from build123d import *

# Parameters (mm, degrees)
F0_R     = 11.5
F1_DEPTH = 11
F2_R     = 11.5
F3_DEPTH = 3
F6_DEPTH = 10


# Not quite as in the source:
# - a fillet or chamfer that OpenCascade refuses, or shapes differently, is made with other operations: its cross-section is extruded or revolved along the edge and cut away or added


with BuildPart() as f1:
    # F0 (on Top) → F1 (new body)
    with BuildSketch(Plane.XY):
        Circle(F0_R)
        Polygon((9.5, 1.5), (9.5, -1.5), (1.5, -1.5), (1.5, -9.5), (-1.5, -9.5), (-1.5, -1.5), (-9.5, -1.5), (-9.5, 1.5), (-1.5, 1.5), (-1.5, 9.5), (1.5, 9.5), (1.5, 1.5), align=None, mode=Mode.SUBTRACT)
    extrude(amount=F1_DEPTH)

    # F2 (on face) → F3 (join)
    with BuildSketch(Plane.XY.offset(11)):
        Circle(F2_R)
        Polygon((1.5, 1.5), (9.5, 1.5), (9.5, -1.5), (1.5, -1.5), (1.5, -9.5), (-1.5, -9.5), (-1.5, -1.5), (-9.5, -1.5), (-9.5, 1.5), (-1.5, 1.5), (-1.5, 9.5), (1.5, 9.5), align=None, mode=Mode.SUBTRACT)
    extrude(amount=F3_DEPTH)

    # F4: fillet of radius 5 on 1 edges, made by hand

    # F4_s1 → F4_t2 (revolve, cut)
    with BuildSketch(Plane.XZ):
        with BuildLine():
            ThreePointArc((11.5, 9), (10.0355339059, 12.5355339059), (6.5, 14))
            Line((6.5, 14), (11.5, 14))
            Line((11.5, 14), (11.5, 9))
        make_face()
    revolve(axis=Axis((0, 0, 14), (0, 0, 1)), mode=Mode.SUBTRACT)

    # F5 (on face) → F6 (join, symmetric)
    with BuildSketch(Plane.XY.offset(14)):
        with BuildLine():
            ThreePointArc((2, -1.5), (2.3717082451, -0.790569415), (2.5, 0))
            ThreePointArc((2.5, 0), (2.3717082451, 0.790569415), (2, 1.5))
            Line((2, 1.5), (1.5, 1.5))
            Line((1.5, 1.5), (1.5, 2))
            ThreePointArc((1.5, 2), (0, 2.5), (-1.5, 2))
            Line((-1.5, 2), (-1.5, 1.5))
            Line((-1.5, 1.5), (-2, 1.5))
            ThreePointArc((-2, 1.5), (-2.5, 0), (-2, -1.5))
            Line((-2, -1.5), (-1.5, -1.5))
            Line((-1.5, -1.5), (-1.5, -2))
            ThreePointArc((-1.5, -2), (0, -2.5), (1.5, -2))
            Line((1.5, -2), (1.5, -1.5))
            Line((1.5, -1.5), (2, -1.5))
        make_face()
        with BuildLine():
            ThreePointArc((1.5, -2), (1.767766953, -1.767766953), (2, -1.5))
            Line((2, -1.5), (1.5, -1.5))
            Line((1.5, -1.5), (1.5, -2))
        make_face()
        with BuildLine():
            Line((-1.5, 1.5), (-1.5, 2))
            ThreePointArc((-1.5, 2), (-1.767766953, 1.767766953), (-2, 1.5))
            Line((-2, 1.5), (-1.5, 1.5))
        make_face()
        with BuildLine():
            ThreePointArc((-2, -1.5), (-1.767766953, -1.767766953), (-1.5, -2))
            Line((-1.5, -2), (-1.5, -1.5))
            Line((-1.5, -1.5), (-2, -1.5))
        make_face()
    extrude(amount=F6_DEPTH, both=True)


solid = f1.part
Model file for the job. Use its own axes, mm. A direction names the side the tool comes from. Coordinates: 2 decimals unless noted, no trailing zeros. Write each loop counter-clockwise with the first axis right and the second up, starting at its lowest first coordinate (ties: lowest second). Pieces come first, ordered by that corner, then holes. Notation, with made-up numbers: (5, -19.5) -> (39, -19.5) arc R16 ccw to (39, -9.5) -> close; hole circle Ø4 at (52.5, -30). An arc over 180 degrees is marked (long way). One line per item, written item: value. Start each with the question number.
1) Probe probe 1 along Y at (x, z) = (-0.5, 6.25); probe 2 along Z at (x, y) = (5.5, -4); probe 3 along X at (y, z) = (7, 11.75). List the from-to ranges inside material, lowest first.
2) Slice it at A-A on x = 0. Write the cut outline in (y, z), then the cut area to 3 significant figures.
3) Pull direction Y, two halves, no side cores. Call faces 1 (the face through (-1.5, 11.4, 4.4)), 2 (the face through (-3, 3, 14)), 3 (the face through (-6, 1.5, 7)): +Y half, -Y half, draft (parallel to the pull), parting line (faces both ways), or undercut.
4) Flat gauge pins, fed straight in: pin 1 Ø4 at (x, y) = (-1.5, 1.5) entering from -Z; pin 2 Ø4 at (y, z) = (5, 9.5) entering from +X; pin 3 Ø2.5 at (y, z) = (-7, 7) entering from -X; pin 4 Ø5 at (x, y) = (7.5, -1.5) entering from +Z. Where does each tip first touch, or does it go through?
5) Which spindle directions (+Z, -Z, +X, -X, +Y, -Y) get a long thin tool onto all of the face, cutting with end or side? Do faces 4 (the face through (-3, -3, 14)), 5 (the face through (3, -3, 14)), 6 (the face through (0, -9.5, 6)), 7 (the face through (3, 3, 14)). Say none if no direction does.
6) Slice it at B-B on z = 18.25. Write the cut outline in (x, y).
Answers follow:
1. probe 1: -11.49 to -9.5, -2.45 to 2.45, 9.5 to 11.49
1. probe 2: 0 to 13.99
1. probe 3: -8.06 to -1.5, 1.5 to 8.06
2. outline: (-11.5, 0) -> (-9.5, 0) -> (-9.5, 13) arc R5 ccw to (-11.5, 9) -> close; (-2.5, 4) -> (2.5, 4) -> (2.5, 24) -> (-2.5, 24) -> close; (9.5, 0) -> (11.5, 0) -> (11.5, 9) arc R5 ccw to (9.5, 13) -> close
2. area: 147 mm2
3. face 1: parting line
3. face 2: draft
3. face 3: undercut
4. pin 1: z = 0
4. pin 2: x = 11.09
4. pin 3: x = -9.96
4. pin 4: z = 14
5. face 4: +Z, -X, -Y
5. face 5: +Z, +X, -Y
5. face 6: +Z, -Z
5. face 7: +Z, +X, +Y
6. outline: (1.5, 1.5) -> (1.5, 2) arc R2.5 ccw (long way) to (2, 1.5) -> close
